Design review of the part shown in the three views and the two pictorial views. Dimensions are in mm from the part's minimum x, y and z. A direction names the side the tool comes from. Coordinates: 2 decimals unless noted, no trailing zeros. Loops run counter-clockwise (first coordinate to the right, second up) from the corner with the lowest first, then second, coordinate; pieces in that order, holes last. Notation, with made-up numbers: (73.25, 4) -> (96.25, 4) arc R37 ccw to (96.25, 43) -> close; hole circle Ø1 at (56, 87.25). An arc over 180 degrees is marked (long way). Answer in a Markdown table with one row per item.
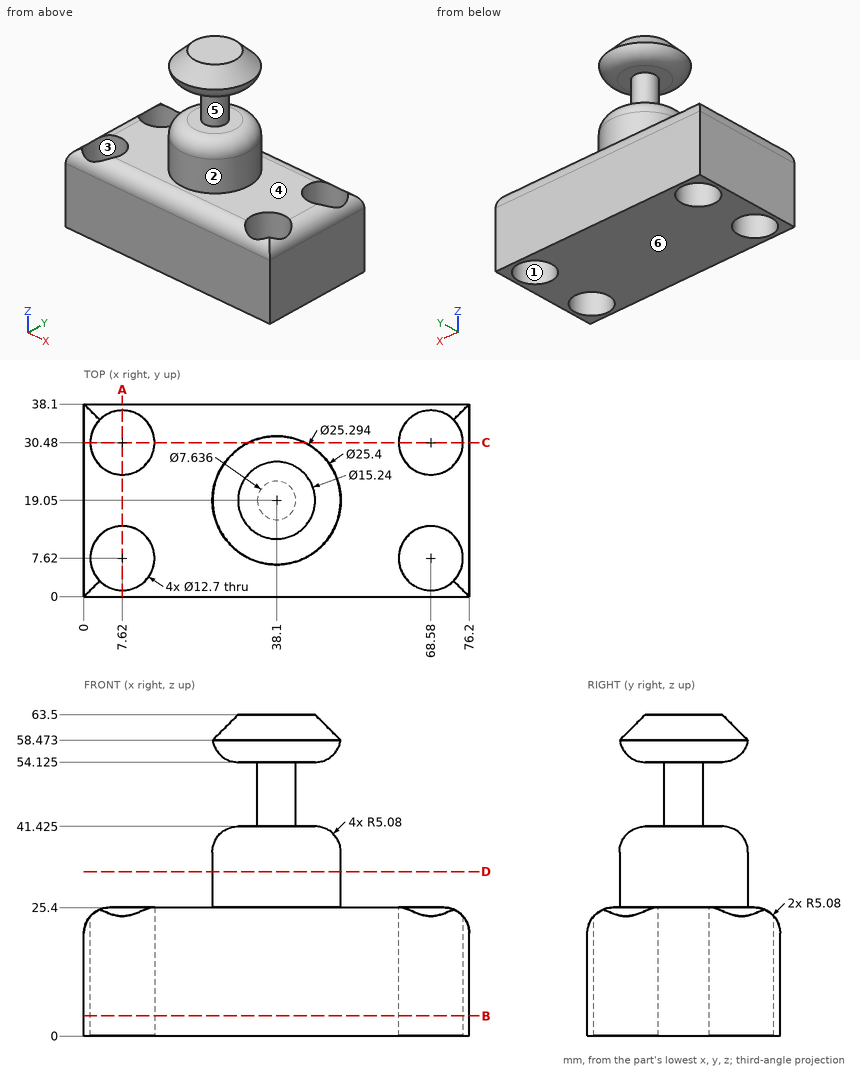
Item 1: Take a section at B-B, the plane z = 4. State the section outline as (x, y) points.
Worked answers:
| item | result |
|---|---|
| outline | (0, 0) -> (76.2, 0) -> (76.2, 38.1) -> (0, 38.1) -> close; hole circle Ø12.7 at (7.62, 7.62); hole circle Ø12.7 at (7.62, 30.48); hole circle Ø12.7 at (68.58, 7.62); hole circle Ø12.7 at (68.58, 30.48) |
Item 2: Take a section at D-D, the plane z = 32.5. State the section outline as (x, y) points, and give its area (3 significant figures).
Worked answers:
| item | result |
|---|---|
| outline | circle Ø25.4 at (38.1, 19.05) |
| area | 507 mm² |
Item 3: For L1, parallel to Y at x = 7.62, z = 5.5; L2, parallel to X at y = 30, z = 13; L3, parallel to X at y = 7, z = 17, list the stretches that pass through material, from the lowest coordinate up.
Worked answers:
| item | result |
|---|---|
| L1 | 0 to 1.27, 13.97 to 24.13, 36.83 to 38.1 |
| L2 | 0 to 1.29, 13.95 to 62.25, 74.91 to 76.2 |
| L3 | 0 to 1.3, 13.94 to 62.26, 74.9 to 76.2 |
Item 4: The part is to be moulded in two halves that separate along Z. For the marked faces 3, 4, 5 and 6, say which applies: +Z half, -Z half, draft (parallel to the pull), parting line (faces both ways), or undercut.
Worked answers:
| item | result |
|---|---|
| face 3 | draft |
| face 4 | +Z half |
| face 5 | undercut |
| face 6 | -Z half |
Item 5: Insertion check: pin 1 (5 mm diameter, centred on x = 46.5, y = 34, fed in from +Z); pin 2 (12 mm diameter, centred on x = 34, z = 33.5, fed in from -Y); pin 3 (14 mm diameter, centred on x = 53, y = 21, fed in from +Z). Each pin has a flat end and moves straight along its axis. Give the tip position at first contact, or say it passes through.
Worked answers:
| item | result |
|---|---|
| pin 1 | z = 25.4 |
| pin 2 | y = 6.35 |
| pin 3 | z = 63.09 |
Item 6: Take a section at C-C, the plane y = 30.48. Count the separate pieces of the cut face and the enclosed holes in it, and give its area (3 significant figures).
Worked answers:
| item | result |
|---|---|
| separate pieces | 4 |
| enclosed holes | 0 |
| area | 1,460 mm² |
Item 7: For the marked faces 1 and 2, list the 3-axis set-ups (+Z, -Z, +X, -X, +Y, -Y) from which the entire face can be reached by the end or side of a thin tool; tool diameter is ignored.
Worked answers:
| item | result |
|---|---|
| face 1 | +Z, -Z |
| face 2 | +Z |
Item 8: Take a section at A-A, the plane x = 7.62. State the section outline as (y, z) points.
Worked answers:
| item | result |
|---|---|
| outline | (0, 0) -> (1.27, 0) -> (1.27, 23.68) arc R5.08 ccw to (0, 20.32) -> close; (13.97, 0) -> (24.13, 0) -> (24.13, 25.4) -> (13.97, 25.4) -> close; (36.83, 0) -> (38.1, 0) -> (38.1, 20.32) arc R5.08 ccw to (36.83, 23.68) -> close |
